Source: CAD feature listing. Evaluate the final solid. Frame: model axes, mm. A direction names the side the tool comes from. Give positions to 0.01 mm unless a question says otherwise; leave off trailing zeros. Loops run counter-clockwise (first coordinate to the right, second up) from the corner with the lowest first, then second, coordinate; pieces in that order, holes last. Notation, with made-up numbers: (52.5, 20) -> (108.5, 20) arc R21 cw to (108.5, 55) -> close; hole circle Ø9 at (71.25, 21). An arc over 180 degrees is marked (long way). Put each result on its own line as item: value.
```python
from build123d import *

# Parameters (mm, degrees)
ESQUISSE1_W             = 8.6
ESQUISSE1_H             = 11.2
BOSS_EXTRU_1_DEPTH      = 18
COQUE1_T                = -1
ESQUISSE2_R             = 3
ENL_V_MAT_EXTRU_1_DEPTH = 20
CONG_2_R                = 0.5


with BuildPart() as part:
    # Esquisse1 → Boss.-Extru.1 (new body)
    with BuildSketch(Plane.XY):
        with Locations((-0.468112778, -1.663701506)):
            Rectangle(ESQUISSE1_W, ESQUISSE1_H)
    extrude(amount=BOSS_EXTRU_1_DEPTH)

    # Coque1
    coque1_openings = [part.faces().sort_by_distance(p)[0] for p in [
        (-0.468112778, -1.663701506, 18),
    ]]
    offset(amount=COQUE1_T, openings=coque1_openings, kind=Kind.INTERSECTION)

    # Esquisse2 → Enlèv. mat.-Extru.1 (cut)
    with BuildSketch(Plane(origin=(3.831887222, 0, 0), x_dir=(0, 0, -1), z_dir=(1, 0, 0))):
        with BuildLine():
            ThreePointArc((-1, 3.936298494), (-0.267949192, 3.204247687), (0, 2.204247687))
            Line((0, 2.204247687), (0, 3.936298494))
            Line((0, 3.936298494), (-1, 3.936298494))
        make_face()
        with BuildLine():
            Line((-1, -7.263701506), (0, -7.263701506))
            Line((0, -7.263701506), (0, -5.531650698))
            ThreePointArc((0, -5.531650698), (-0.267949192, -6.531650698), (-1, -7.263701506))
        make_face()
        with Locations((-11, -1.663701506)):
            Circle(ESQUISSE2_R)
    extrude(amount=-ENL_V_MAT_EXTRU_1_DEPTH, mode=Mode.SUBTRACT)

    # Congé2
    cong_2_edges = [part.edges().sort_by_distance(p)[0] for p in [
        (-0.468112778, 3.936298494, 18),
        (-0.468112778, 3.936298494, 1),
        (-0.468112778, -7.263701506, 1),
        (-4.768112778, 3.936298494, 9.5),
        (3.831887222, 3.936298494, 9.5),
        (3.831887222, -7.263701506, 9.5),
        (-4.768112778, -7.263701506, 9.5),
        (-0.468112778, -7.263701506, 18),
    ]]
    fillet(cong_2_edges, radius=CONG_2_R)


solid = part.part
```
(1) Line query: probe 1 along X at (y, z) = (1.5, 10.5); probe 2 along Y at (x, z) = (-3.95, 11); probe 3 along Y at (x, z) = (1.25, 14). Output: solid intervals per line, ascending. Write a range as from..to.
Calculated:
probe 1: x = -4.77..-3.77, 2.83..3.83
probe 2: y = -7.26..-4.66, 1.34..3.94
probe 3: y = -7.26..-6.26, 2.94..3.94
(2) Reachability of faces 1 (the flat face through (-4, -1, 18)), 2 (the flat face through (-1, -2, 1)) from +Z, -Z, +X, -X, +Y, -Y: full face, straight path, thin tool, end or side. Return the list, or none.
Calculated:
face 1: +Z, +X, -X, +Y, -Y
face 2: +Z
(3) Section D-D on y = -2. Return loops of the section in (x, z), then the cut area to 3 significant figures.
Calculated:
outline: (-4.77, 0) -> (3.83, 0) -> (3.83, 8.02) -> (2.83, 8.02) -> (2.83, 1) -> (-3.77, 1) -> (-3.77, 8.02) -> (-4.77, 8.02) -> close; (-4.77, 13.98) -> (-3.77, 13.98) -> (-3.77, 18) -> (-4.77, 18) -> close; (2.83, 13.98) -> (3.83, 13.98) -> (3.83, 18) -> (2.83, 18) -> close
area: 30.7 mm²
(4) Section A-A on z = 11. Return loops of the section in (x, y), then the cut area to 3 significant figures.
Calculated:
outline: (-4.77, -6.76) arc R0.5 ccw to (-4.27, -7.26) -> (3.33, -7.26) arc R0.5 ccw to (3.83, -6.76) -> (3.83, -4.66) -> (2.83, -4.66) -> (2.83, -6.26) -> (-3.77, -6.26) -> (-3.77, -4.66) -> (-4.77, -4.66) -> close; (-4.77, 1.34) -> (-3.77, 1.34) -> (-3.77, 2.94) -> (2.83, 2.94) -> (2.83, 1.34) -> (3.83, 1.34) -> (3.83, 3.44) arc R0.5 ccw to (3.33, 3.94) -> (-4.27, 3.94) arc R0.5 ccw to (-4.77, 3.44) -> close
area: 23.4 mm²
(5) Section C-C on z = 4. Return loops of the section in (x, y), then the cut area to 3 significant figures.
Calculated:
outline: (-4.77, -6.76) arc R0.5 ccw to (-4.27, -7.26) -> (3.33, -7.26) arc R0.5 ccw to (3.83, -6.76) -> (3.83, 3.44) arc R0.5 ccw to (3.33, 3.94) -> (-4.27, 3.94) arc R0.5 ccw to (-4.77, 3.44) -> close; hole (-3.77, -6.26) -> (2.83, -6.26) -> (2.83, 2.94) -> (-3.77, 2.94) -> close
area: 35.4 mm²
(6) Draft query along Y for faces 3 (the flat face through (-1, -7.264, 9)), 4 (the flat face through (3.832, -2, 7)), 5 (the cylindrical face through (-0.408, 3.143, 0.234)), 6 (the cylindrical face through (-4.261, -1.532, 13.997)). Return one class per face: released by +Y, released by -Y, zero draft, split by the parting line, or undercut.
Calculated:
face 3: released by -Y
face 4: zero draft
face 5: released by +Y
face 6: undercut
(7) Section B-B on x = 1. Return loops of the section in (y, z).
Calculated:
outline: (-7.26, 1.14) arc R0.5 ccw to (-7.17, 0.86) arc R2 ccw to (-5.53, 0) -> (2.2, 0) arc R2 ccw to (3.85, 0.86) arc R0.5 ccw to (3.94, 1.14) -> (3.94, 17.5) arc R0.5 ccw to (3.44, 18) -> (2.94, 18) -> (2.94, 1) -> (-6.26, 1) -> (-6.26, 18) -> (-6.76, 18) arc R0.5 ccw to (-7.26, 17.5) -> close
